from build123d import *

# Parameters (mm, degrees)
BOSS_EXTRUDE1_DEPTH      = 12.7
BOSS_EXTRUDE1_DEPTH_BACK = 0.364929482
SKETCH1_W                = 76.2
SKETCH1_H                = 7.62
SKETCH14_W               = 38.1
SKETCH14_H               = 7.62
CUT_EXTRUDE5_DEPTH       = 19.558
BOSS_EXTRUDE2_START      = -8
SKETCH15_W               = 2.54
SKETCH15_H               = 21.3868
SKETCH15_W_2             = 3.175
SKETCH15_H_2             = 5.842
BOSS_EXTRUDE2_DEPTH      = 5.08
FILLET1_R                = 7.62
FILLET2_R                = 1.27
SKETCH17_W               = 3.556
SKETCH17_H               = 3.014496912
BOSS_EXTRUDE3_DEPTH      = 5.08
SKETCH18_W               = 20.32
SKETCH18_H               = 66
BOSS_EXTRUDE4_DEPTH      = 10.16
SKETCH19_W               = 17.109306796
SKETCH19_H               = 60.063536248
CUT_EXTRUDE14_DEPTH      = 8.89
FILLET3_R                = 4.92


with BuildPart() as part:
    # Sketch1 → Boss-Extrude1 (new, two sides: drawn at the far end of the back side and taken through both)
    with BuildSketch(Plane(origin=(0, 0, 0), x_dir=(1, 0, 0), z_dir=(0, 1, 0)).offset(-BOSS_EXTRUDE1_DEPTH_BACK)):
        Rectangle(SKETCH1_W, SKETCH1_H)
    extrude(amount=BOSS_EXTRUDE1_DEPTH + BOSS_EXTRUDE1_DEPTH_BACK)

    # Sketch14 → Cut-Extrude5 (cut)
    with BuildSketch(Plane(origin=(0, 12.7, 0), x_dir=(1, 0, 0), z_dir=(0, 1, 0))):
        with Locations((19.05, 0)):
            Rectangle(SKETCH14_W, SKETCH14_H)
    extrude(amount=-CUT_EXTRUDE5_DEPTH, mode=Mode.SUBTRACT)

    # Sketch15 → Boss-Extrude2 (add)
    with BuildSketch(Plane(origin=(0, 12.7, 0), x_dir=(1, 0, 0), z_dir=(0, 1, 0)).offset(BOSS_EXTRUDE2_START)):
        with Locations((-3.048, -14.5034)):
            Rectangle(SKETCH15_W, SKETCH15_H)
        with BuildLine():
            ThreePointArc((-8.89, -25.1968), (-6.604, -31.907368859), (-4.318, -25.1968))
            Line((-4.318, -25.1968), (-1.778, -25.1968))
            ThreePointArc((-1.778, -25.1968), (-6.604, -33.827245709), (-11.43, -25.1968))
            Line((-11.43, -25.1968), (-11.43, -8.4836))
            Line((-11.43, -8.4836), (-8.89, -8.4836))
            Line((-8.89, -8.4836), (-8.89, -25.1968))
        make_face()
        with Locations((-13.0175, -16.4592)):
            Rectangle(SKETCH15_W_2, SKETCH15_H_2)
    extrude(amount=-BOSS_EXTRUDE2_DEPTH)

    # Fillet1
    fillet1_edges = [part.edges().sort_by_distance(p)[0] for p in [
        (-11.43, 2.16, 25.1968),
        (-1.778, 2.16, 25.1968),
        (-8.89, 2.16, 25.1968),
        (-4.318, 2.16, 25.1968),
    ]]
    fillet(fillet1_edges, radius=FILLET1_R)

    # Fillet2
    fillet2_edges = [part.edges().sort_by_distance(p)[0] for p in [
        (-11.43, 2.16, 19.3802),
        (-14.605, 2.16, 19.3802),
        (-14.605, 2.16, 13.5382),
        (-11.43, 2.16, 13.5382),
        (-8.89, 2.16, 8.4836),
        (-11.43, 2.16, 8.4836),
    ]]
    fillet(fillet2_edges, radius=FILLET2_R - 0.0001)  # a hair under: the kernel refuses the full size

    # Mirror1: part across plane


with BuildPart() as part_1:
    add(part.part)
    add(part.part.mirror(Plane(origin=(0, -6.858, -3.81), x_dir=(0, 0, 1), z_dir=(-1, 0, 0))))

    # Sketch17 → Boss-Extrude3 (add)
    with BuildSketch(Plane(origin=(0, 4.7, 0), x_dir=(1, 0, 0), z_dir=(0, 1, 0))):
        with Locations((0, -8.490791694)):
            Rectangle(SKETCH17_W, SKETCH17_H)
        with Locations((0, -18.593429993)):
            Rectangle(SKETCH17_W, SKETCH17_H)
    extrude(amount=-BOSS_EXTRUDE3_DEPTH)

    # Sketch18 → Boss-Extrude4 (add)
    with BuildSketch(Plane(origin=(0, 12.7, 0), x_dir=(1, 0, 0), z_dir=(0, 1, 0))):
        with Locations((0, -29.19)):
            Rectangle(SKETCH18_W, SKETCH18_H)
    extrude(amount=BOSS_EXTRUDE4_DEPTH)

    # Sketch19 → Cut-Extrude14 (cut)
    with BuildSketch(Plane(origin=(0, 22.86, 0), x_dir=(1, 0, 0), z_dir=(0, 1, 0))):
        with Locations((0, -29.19)):
            Rectangle(SKETCH19_W, SKETCH19_H)
    extrude(amount=-CUT_EXTRUDE14_DEPTH, mode=Mode.SUBTRACT)

    # Fillet3
    fillet3_edges = [part_1.edges().sort_by_distance(p)[0] for p in [
        (0, 12.7, 3.81),
    ]]
    fillet(fillet3_edges, radius=FILLET3_R)


solid = part_1.part
For this review, take the finished solid that the model builds, in its own axes (mm). A direction names the side the tool comes from. Round coordinates to 2 decimals unless told otherwise and drop trailing zeros. Order: outer loops, then holes, each group sorted by start corner. A loop starts at its lowest first (then second) coordinate and runs counter-clockwise, first axis right, second up. Notation, with made-up numbers: M 31,-14 L 69,-14 A28 ccw 69,16 Z; hole C 84,-35 d5. An arc over 180 degrees is marked long. Write each question's results on one line, items separated by ' | '. Start each with the question number.
1. Add section B-B (y = 17.5). State the section outline as (x, z) points, then the cut area to 3 significant figures.
2. Clearance check with flat-ended pins moving along their axes: pin 1 Ø1.7 at (y, z) = (1.5, 17) entering from -X (3 decimals); pin 2 Ø1 at (y, z) = (1.5, 5) entering from +X; pin 3 Ø12 at (y, z) = (13, 38) entering from -X; pin 4 Ø5 at (x, y) = (-21.5, 17) entering from +Z. State where each tip first meets the part, or that it passes through.
3. Tool access review of faces 1 (the face through (24, 12.7, 0)), 2 (the face through (0, 2, 17.086)), 3 (the face through (0, 18, 59.222)): name each direction out of +Z, -Z, +X, -X, +Y, -Y from which nothing blocks a thin tool from reaching the whole face with its end or side.
4. To check wall thickness, follow L1, parallel to X at y = 3.5, z = 5; L2, parallel to X at y = 1.75, z = 20; L3, parallel to X at y = 19.25, z = 43.5. State the ranges of each line that lie inside material, in increasing order. Write a range as [from, to].
5. Add section D-D (y = 6). State the section outline as (x, z) points, then the cut area to 3 significant figures.
6. Add section C-C (z = 46). State the section outline as (x, y) points, then the cut area to 3 significant figures.
7. Draft analysis for pull direction Z (two halves, no side actions). For faces 4 (the face through (-11.43, 2, 11)), 5 (the face through (-10.16, 17, 30)), state which applies: pulls with the +Z half, pulls with the -Z half, needs draft (parallel to the pull), parting line crosses it, or undercut.
8. Add section A-A (z = 11). State the section outline as (x, y) points, then the cut area to 3 significant figures.
Output values:
1) outline: M -10.16,-3.81 L 10.16,-3.81 L 10.16,62.19 L -10.16,62.19 Z; hole M -8.55,-0.84 L 8.55,-0.84 L 8.55,59.22 L -8.55,59.22 Z | area: 313 mm^2
2) pin 1: x = -14.605 | pin 2: x = 4.32 | pin 3: x = -10.16 | pin 4: through
3) face 1: +Z, -Z, +X, +Y | face 2: -Y | face 3: +Y
4) L1: [-4.32, -1.78], [1.78, 4.32] | L2: [-11.61, -8.89], [-4.32, 4.32], [8.89, 11.61] | L3: [-10.16, -8.55], [8.55, 10.16]
5) outline: M -38.1,-3.81 L 38.1,-3.81 L 38.1,3.81 L -38.1,3.81 Z | area: 581 mm^2
6) outline: M -10.16,12.7 L 10.16,12.7 L 10.16,22.86 L 8.55,22.86 L 8.55,13.97 L -8.55,13.97 L -8.55,22.86 L -10.16,22.86 Z | area: 54.3 mm^2
7) face 4: undercut | face 5: needs draft
8) outline: M -11.43,-0.38 L -8.89,-0.38 L -8.89,4.7 L -11.43,4.7 Z; M -10.16,12.7 L 10.16,12.7 L 10.16,22.86 L 8.55,22.86 L 8.55,13.97 L -8.55,13.97 L -8.55,22.86 L -10.16,22.86 Z; M -4.32,-0.38 L -1.78,-0.38 L -1.78,4.7 L -4.32,4.7 Z; M 1.78,-0.38 L 4.32,-0.38 L 4.32,4.7 L 1.78,4.7 Z; M 8.89,-0.38 L 11.43,-0.38 L 11.43,4.7 L 8.89,4.7 Z | area: 106 mm^2
